```python
from build123d import *

# Parameters (mm, degrees)
F1_DEPTH = 25.4


with BuildPart() as f1:
    # F0 (on Top) → F1 (new body)
    with BuildSketch(Plane.XY):
        Polygon((-7.199717, -15.923513), (-1.659717, -15.923513), (67.800283, -15.923513), (67.800283, -2.923513), (-7.199717, -2.923513), (-7.199717, -12.923513), align=None)
        with BuildLine():
            Line((62.260283, -12.923513), (-1.659717, -12.923513))
            ThreePointArc((-1.659717, -12.923513), (-3.455768, -12.179564), (-4.199717, -10.383513))
            Line((-4.199717, -10.383513), (-4.199717, -8.463513))
            ThreePointArc((-4.199717, -8.463513), (-3.455768, -6.667462), (-1.659717, -5.923513))
            Line((-1.659717, -5.923513), (62.260283, -5.923513))
            ThreePointArc((62.260283, -5.923513), (64.056334, -6.667462), (64.800283, -8.463513))
            Line((64.800283, -8.463513), (64.800283, -10.383513))
            ThreePointArc((64.800283, -10.383513), (64.056334, -12.179564), (62.260283, -12.923513))
        make_face(mode=Mode.SUBTRACT)
    extrude(amount=F1_DEPTH)


solid = f1.part
```
Work out the finished part from the listing and answer in its coordinate system (mm). A direction names the side the tool comes from. Round coordinates to 2 decimals unless told otherwise and drop trailing zeros. Write each loop counter-clockwise with the first axis right and the second up, starting at its lowest first coordinate (ties: lowest second). Pieces come first, ordered by that corner, then holes. Notation, with made-up numbers: (12.25, 72.25) - (68.25, 72.25) arc R24 cw to (68.25, 109.25) - close; hole circle Ø6 at (67, 4). An arc over 180 degrees is marked (long way). Return JSON: item names as keys, results as strings. Group by question number.
Q1. The part is cut by section A-A on x = 52.5. Write down the section's boundary in (y, z).
Q2. The mould has two halves that part along Y. Classify faces 3 (the flat face through (30, -15.924, 13)), 4 (the flat face through (-7.2, -9, 13)), 5 (the cylindrical face through (-3.48, -6.69, 12.52)), 6 (the flat face through (64.8, -9, 13)): released by +Y, released by -Y, zero draft, split by the parting line, or undercut.
Q3. For faces 1 (the flat face through (67.8, -10, 13)), 2 (the flat face through (-4.2, -9, 13)), determine the directions among +Z, -Z, +X, -X, +Y, -Y from which every point of the face is accessible in a straight line to the end or side of a thin tool.
Q4. The part is cut by section C-C on y = -7.5. Write down the section's boundary in (x, z).
Q5. Find the intervals of material crossed by L1, parallel to Y at x = 7.5, z = 13.5; L2, parallel to X at y = -7.25, z = 8; L3, parallel to X at y = -8, z = 24.25, in increasing order.
Q6. The part is cut by section B-B on z = 9.5. Write down the section's boundary in (x, y).
Q7. This flat-tipped pin is pushed along its axis until it touches: pin 1 Ø1.5 at (x, y) = (20.5, -8.5) entering from -Z. Where does it stop, or does it pass through?
Solved:
{
 "1": {"outline": "(-15.92, 0) - (-12.92, 0) - (-12.92, 25.4) - (-15.92, 25.4) - close; (-5.92, 0) - (-2.92, 0) - (-2.92, 25.4) - (-5.92, 25.4) - close"},
 "2": {"face 3": "released by -Y", "face 4": "zero draft", "face 5": "undercut", "face 6": "undercut"},
 "3": {"face 1": "+Z, -Z, +X, +Y, -Y", "face 2": "+Z, -Z"},
 "4": {"outline": "(-7.2, 0) - (-4.01, 0) - (-4.01, 25.4) - (-7.2, 25.4) - close; (64.61, 0) - (67.8, 0) - (67.8, 25.4) - (64.61, 25.4) - close"},
 "5": {"L1": "-15.92 to -12.92, -5.92 to -2.92", "L2": "-7.2 to -3.89, 64.49 to 67.8", "L3": "-7.2 to -4.16, 64.76 to 67.8"},
 "6": {"outline": "(-7.2, -15.92) - (67.8, -15.92) - (67.8, -2.92) - (-7.2, -2.92) - close; hole (-4.2, -10.38) arc R2.54 ccw to (-1.66, -12.92) - (62.26, -12.92) arc R2.54 ccw to (64.8, -10.38) - (64.8, -8.46) arc R2.54 ccw to (62.26, -5.92) - (-1.66, -5.92) arc R2.54 ccw to (-4.2, -8.46) - close"},
 "7": {"pin 1": "through"}
}
